from build123d import *

# Parameters (mm, degrees)
FILLET1_R          = 2
SKETCH2_R          = 5.775
EXTRUDE1_DEPTH     = 1
SKETCH3_R          = 2.375
EXTRUDE2_DEPTH     = 2
SKETCH4_R          = 0.435
EXTRUDE3_DEPTH     = 0.5
CIRPATTERN1_COUNT  = 10
SKETCH5_R          = 1.9
CUT_EXTRUDE1_DEPTH = 30.83705763
CIRPATTERN2_COUNT  = 8
SKETCH6_R          = 1.63
CUT_EXTRUDE2_DEPTH = 10.9125


with BuildPart() as part:
    # Sketch1 → Revolve1 (revolve)
    with BuildSketch(Plane.XY, mode=Mode.PRIVATE) as revolve1_sk:
        with BuildLine():
            Line((9.5, 0), (0, 0))
            Line((0, 0), (0, 3.1))
            Line((0, 3.1), (7.5, 3.1))
            Line((7.5, 3.1), (7.5, 14.5))
            Line((7.5, 14.5), (7, 15))
            Line((7, 15), (7, 16.677124344))
            ThreePointArc((7, 16.677124344), (8.5, 20), (10, 16.677124344))
            Line((10, 16.677124344), (10, 15))
            Line((10, 15), (9.5, 14.5))
            Line((9.5, 14.5), (9.5, 0))
        make_face()
    revolve(revolve1_sk.sketch.rotate(Axis((0, 0, 0), (1, 0, 0)), 90), axis=Axis((0, 0, 0), (1, 0, 0)))

    # Fillet1
    fillet1_edges = [part.edges().sort_by_distance(p)[0] for p in [
        (7, 0, -16.677124344),
        (10, 0, -16.677124344),
    ]]
    fillet(fillet1_edges, radius=FILLET1_R)

    # Sketch2 → Extrude1 (add)
    with BuildSketch(Plane(origin=(9.5, 0, 0), x_dir=(0, 0, -1), z_dir=(1, 0, 0))):
        with Locations(Location((0, 0, 0), (0, 0, 180))):
            Circle(SKETCH2_R)
    extrude(amount=EXTRUDE1_DEPTH)

    # Sketch3 → Extrude2 (add)
    with BuildSketch(Plane(origin=(10.5, 0, 0), x_dir=(0, 0, -1), z_dir=(1, 0, 0))):
        Circle(SKETCH3_R)
    extrude(amount=EXTRUDE2_DEPTH)

    # Sketch4 → Extrude3 (add)
    with BuildSketch(Plane(origin=(10.5, 0, 0), x_dir=(0, 0, -1), z_dir=(1, 0, 0))):
        with Locations((0, 4)):
            Circle(SKETCH4_R)
    extrude3 = extrude(amount=EXTRUDE3_DEPTH)

    # CirPattern1: Extrude3 ×10 about axis
    cirpattern1_axis = Axis((0, 0, 0), (1, 0, 0))
    for i in range(1, CIRPATTERN1_COUNT):
        add(extrude3.rotate(cirpattern1_axis, i * 360 / CIRPATTERN1_COUNT))

    # Sketch5 → Cut-Extrude1 (cut, through all)
    with BuildSketch(Plane(origin=(9.5, 0, 0), x_dir=(0, 0, -1), z_dir=(1, 0, 0))):
        with Locations((0, 10.1375)):
            Circle(SKETCH5_R)
    cut_extrude1 = extrude(amount=-CUT_EXTRUDE1_DEPTH, mode=Mode.SUBTRACT)

    # CirPattern2: Cut-Extrude1 ×8 about axis
    cirpattern2_axis = Axis((0, 0, 0), (1, 0, 0))
    for i in range(1, CIRPATTERN2_COUNT):
        add(cut_extrude1.rotate(cirpattern2_axis, i * 360 / CIRPATTERN2_COUNT), mode=Mode.SUBTRACT)

    # Sketch6 → Cut-Extrude2 (cut)
    with BuildSketch(Plane.ZY):
        Circle(SKETCH6_R)
    extrude(amount=-CUT_EXTRUDE2_DEPTH, mode=Mode.SUBTRACT)


solid = part.part
Design review of the part built by this model. Coordinates are the model's own, in mm. A direction names the side the tool comes from. Give positions to 0.01 mm unless a question says otherwise; leave off trailing zeros. Loops run counter-clockwise (first coordinate to the right, second up) from the corner with the lowest first, then second, coordinate; pieces in that order, holes last. Notation, with made-up numbers: M 2.25,74 L 25.25,74 A23 cw 25.25,97 Z; hole C 57,31.25 d1. An arc over 180 degrees is marked long. One line per question, with ' | ' between items. Start each with the question number.
1. Insertion check: P1, Ø0.7, axis at y = -3.5, z = -2.5, coming from the +X side; P2, Ø1, axis at x = 8, y = -11.5, coming from the -Z side; P3, Ø1.5, axis at x = 7.5, z = -10.5, coming from the -Y side. Each pin has a flat end and moves straight along its axis. Give the tip position at first contact, or say it passes through.
2. The part is to be moulded in two halves that separate along Z. For faces 4 (the face through (12.5, 0, 0)), 5 (the face through (10.746, -1.308, -3.375)), say which applies: released by +Z, released by -Z, zero draft, split by the parting line, or undercut.
3. Add section B-B (y = 0). Give the number of separate pieces and of enclosed holes in the cut face, plus the area to 3 significant figures.
4. For faces 1 (the face through (11, -3.2, -2.4)), 2 (the face through (3.802, -0.931, 2.957)), 3 (the face through (10.746, -3.395, 2.756)), list the 3-axis set-ups (+Z, -Z, +X, -X, +Y, -Y) from which the entire face can be reached by the end or side of a thin tool; tool diameter is ignored.
5. Add section A-A (x = 5.5). Write out the cut boundary in (y, z), plus the area to 3 significant figures.
6. To check wall thickness, follow L1, parallel to Y at x = 7.75, z = 6; L2, parallel to Z at x = 9.75, y = 0.5; L3, parallel to X at y = -3.5, z = 12. State the ranges of each line that lie inside material, in increasing order.
Worked out:
1) P1: stops at x = 11 | P2: stops at z = -16.65 | P3: stops at y = -17.29
2) face 4: zero draft | face 5: undercut
3) separate pieces: 3 | enclosed holes: 0 | area: 110 mm²
4) face 1: +Z, -Z, +X, -Y | face 2: -X | face 3: +X
5) outline: C 0,0 d6.2; hole C 0,0 d3.26 | area: 21.8 mm²
6) L1: y = -18.93 to -8.67, -5.67 to 5.67, 8.67 to 18.93 | L2: z = -19.55 to -14.74, -5.75 to -1.55, 1.55 to 5.75, 14.74 to 19.55 | L3: x = 7.5 to 9.5
